The figure shows three views and two pictorial views of one solid part (mm, origin at its lowest corner). Answer the questions. A direction names the side the tool comes from. Round coordinates to 2 decimals unless told otherwise and drop trailing zeros. Order: outer loops, then holes, each group sorted by start corner. A loop starts at its lowest first (then second) coordinate and runs counter-clockwise, first axis right, second up. Notation, with made-up numbers: (21, 70) -> (71, 70) arc R28 ccw to (71, 104) -> close; hole circle Ø9 at (25, -3). An arc over 180 degrees is marked (long way). One line per item, written item: value. Start each with the question number.
1. Consider line 1 (Y direction, x = 3.65, z = 0.65); line 2 (X direction, y = 4, z = 3.15) (1 decimal); line 3 (Y direction, x = 2.6, z = 2.3). Determine where each line is inside the solid, lowest interval first.
2. Flat-ended cylindrical pins translate along their axes: pin 1 Ø0.9 at (x, z) = (2.5, 2.5) entering from -Y; pin 2 Ø1.5 at (y, z) = (21, 2.5) entering from -X. Find the tip coordinate at first contact, or state that the pin passes through.
3. For the marked faces 1, 2 and 3, determine the directions among +Z, -Z, +X, -X, +Y, -Y from which every point of the face is accessible in a straight line to the end or side of a thin tool.
4. Section B-B (y = 42) is taken. Give the vertices of the cut face in (x, z).
5. Section A-A (y = 28) is taken. Give the vertices of the cut face in (x, z) (1 decimal).
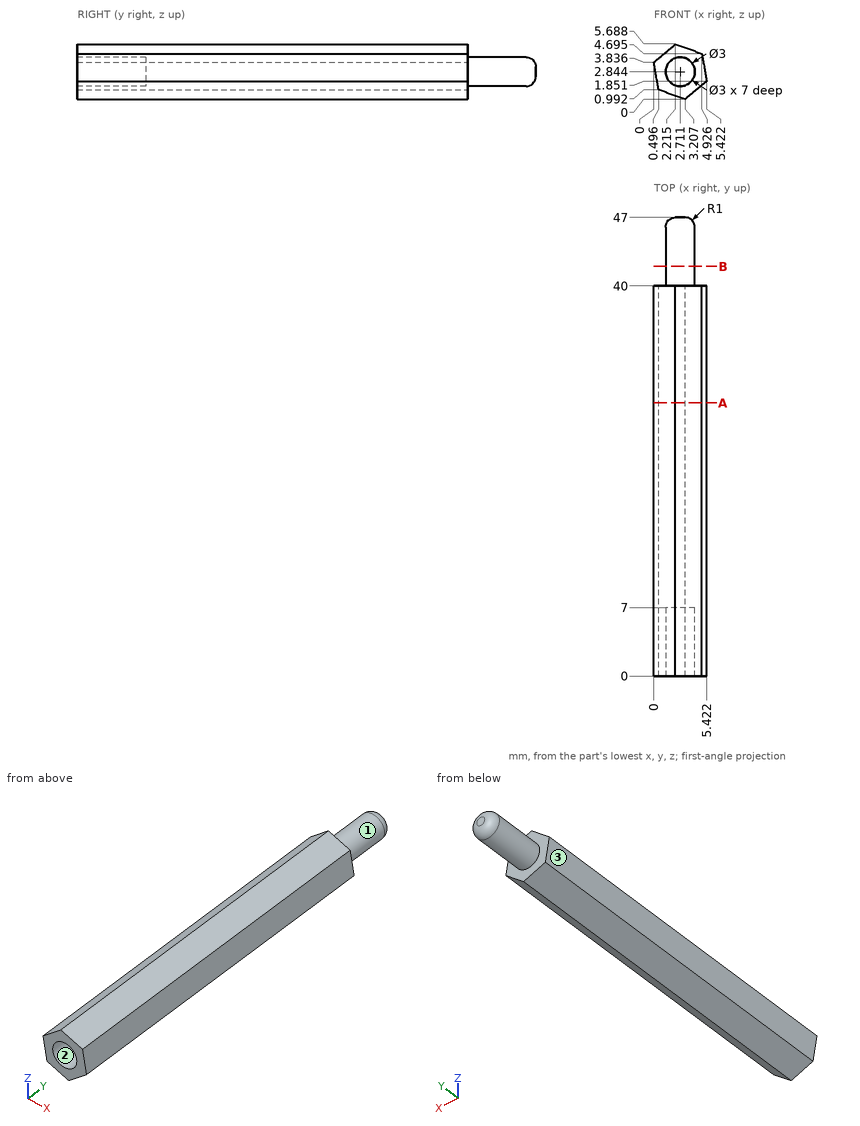
Answer:
1. line 1: 0 to 40
1. line 2: 0.1 to 1.2, 4.2 to 5.2
1. line 3: 7 to 47
2. pin 1: y = 7
2. pin 2: x = 0.1
3. face 1: +Y
3. face 2: -Y
3. face 3: -Z, -X, +Y, -Y
4. outline: circle Ø3 at (2.71, 2.84)
5. outline: (0, 3.8) -> (0.5, 1) -> (3.2, 0) -> (5.4, 1.9) -> (4.9, 4.7) -> (2.2, 5.7) -> close
